Geometry: final body of the model. Coordinates: model frame, mm. Round coordinates to 2 decimals unless told otherwise and drop trailing zeros. Write each loop counter-clockwise with the first axis right and the second up, starting at its lowest first coordinate (ties: lowest second). Pieces come first, ordered by that corner, then holes. Notation, with made-up numbers: M 45.25,4 L 80.25,4 A29 ccw 80.25,40 Z; hole C 1,88.5 d6. An arc over 180 degrees is marked long. Use one line per item in the form item = value. Start each with the question number.
Item 1: Section query B-B (y = -24.5). Return loops of the section in (x, z), and give its area (3 significant figures).
Item 2: Section query C-C (z = 154.5). Return loops of the section in (x, y).
Item 3: Ray query, probe 1 along Z at (x, y) = (0.9, -72); probe 2 along Y at (x, z) = (0.4, 198); probe 3 along Y at (x, z) = (0.25, 20.5). Return the intervals inside material, ascending.
Item 4: Section query A-A (x = 2.5). Return loops of the section in (y, z).
Item 5: Pin query (flat end, axial travel): pin 1 Ø1 at (x, y) = (2, -23.5) entering from -Z; pin 2 Ø1 at (x, z) = (0.5, 72) entering from +Y. Return the tip coordinate at first contact, or that it passes through.
Autodesk Inventor part; units mm, degrees
ref_plane "YZ Plane" through (0, 0, 0) normal (1, 0, 0) x (0, 1, 0)
ref_plane "XZ Plane" through (0, 0, 0) normal (0, 1, 0) x (-1, 0, 0)
ref_plane "XY Plane" through (0, 0, 0) normal (0, 0, 1) x (1, 0, 0)
sketch "スケッチ1" plane through (0, 0, 0) normal (1, 0, 0) x (0, 1, 0)
  line L0 (-90, 263.8963) -> (-90, -36.1037)
  line L1 (-90, -36.1037) -> (90, -100)
  line L2 (-126, 0) -> (126, 0)
  line L3 (0, -172.7793) -> (0, 336.6756)
  line L4 (-90, 263.8963) -> (56.4999, 78.6159)
  line L5 (56.4999, 78.6159) -> (90, -100)
  dimension "d0" = 300
  dimension "d5" = 90
  dimension "d6" = 100
  dimension "d7" = 90
extrude "押し出し1" add sketch "スケッチ1" along normal blind 3
fillet "フィレット1" radius 5 1 edges at (1.5, 90, -100)
properties part number "stay_middle" material "CFRP"
Working result:
q1.outline = M 0,-59.35 L 3,-59.35 L 3,181.06 L 0,181.06 Z
q1.area = 721 mm²
q2.outline = M 0,-90 L 3,-90 L 3,-3.5 L 0,-3.5 Z
q3.probe_1 = -42.49 to 241.13
q3.probe_2 = -90 to -37.9
q3.probe_3 = -90 to 67.4
q4.outline = M -90,-36.1 L 81.81,-97.09 A5 ccw 88.4,-91.46 L 56.5,78.62 L -90,263.9 Z
q5.pin_1 = -59.89
q5.pin_2 = 57.83
